Can you work these out from the drawing? Everything is in mm from the part's minimum corner. Coordinates: 2 decimals unless noted, no trailing zeros. Write each loop counter-clockwise with the first axis right and the second up, starting at its lowest first coordinate (ties: lowest second). Pieces come first, ordered by that corner, then holes. Notation, with made-up numbers: M 64,26.25 L 117,26.25 A24 cw 117,62.25 Z; hole C 89.25,9.5 d8. An arc over 180 degrees is marked long. Write item = value, one per line.
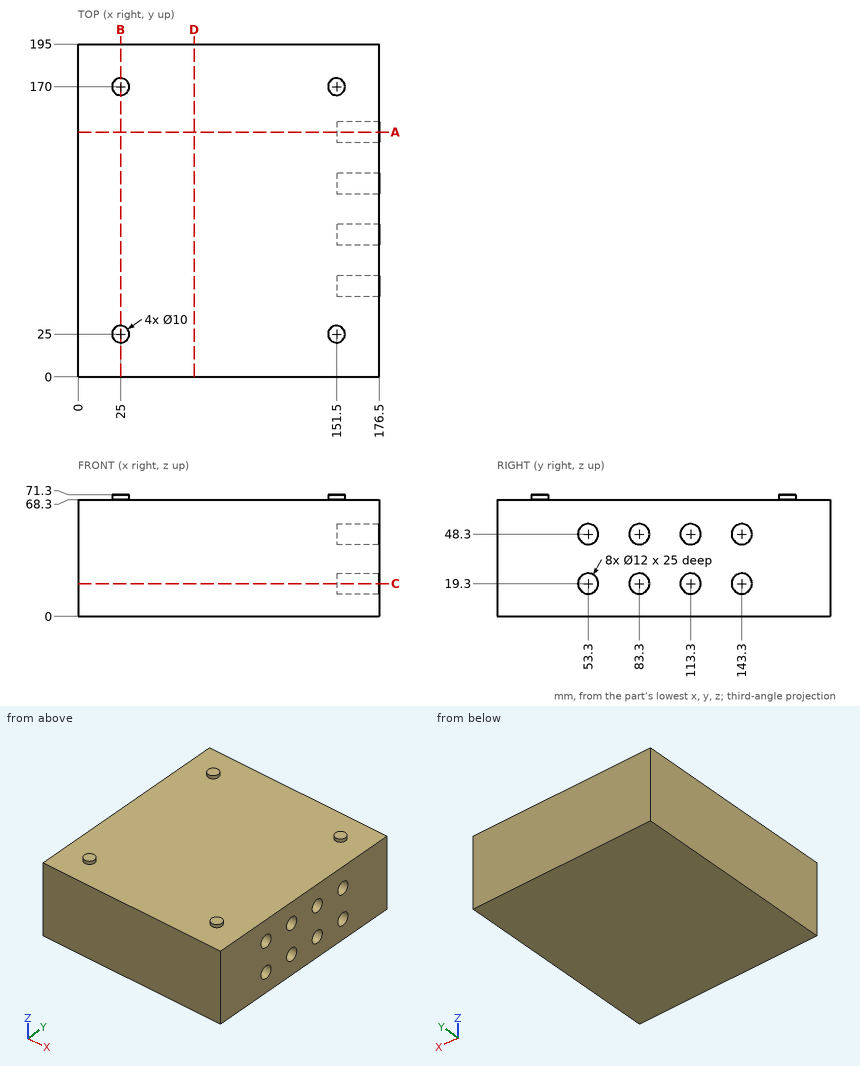
Item 1: Imagine slicing it at B-B (x = 25). Write out the boundary of the cut face in (y, z).
Numbers:
outline = M 0,0 L 195,0 L 195,68.3 L 175,68.3 L 175,71.3 L 165,71.3 L 165,68.3 L 30,68.3 L 30,71.3 L 20,71.3 L 20,68.3 L 0,68.3 Z
Item 2: Imagine slicing it at C-C (z = 19.3). Write out the boundary of the cut face in (x, y).
Numbers:
outline = M 0,0 L 176.5,0 L 176.5,47.3 L 151.5,47.3 L 151.5,59.3 L 176.5,59.3 L 176.5,77.3 L 151.5,77.3 L 151.5,89.3 L 176.5,89.3 L 176.5,107.3 L 151.5,107.3 L 151.5,119.3 L 176.5,119.3 L 176.5,137.3 L 151.5,137.3 L 151.5,149.3 L 176.5,149.3 L 176.5,195 L 0,195 Z
Item 3: Imagine slicing it at A-A (y = 143.3). Write out the boundary of the cut face in (x, z), and give its area (3 significant figures).
Numbers:
outline = M 0,0 L 176.5,0 L 176.5,13.3 L 151.5,13.3 L 151.5,25.3 L 176.5,25.3 L 176.5,42.3 L 151.5,42.3 L 151.5,54.3 L 176.5,54.3 L 176.5,68.3 L 0,68.3 Z
area = 11,500 mm²
Item 4: Imagine slicing it at D-D (x = 68). Write out the boundary of the cut face in (y, z), and give its area (3 significant figures).
Numbers:
outline = M 0,0 L 195,0 L 195,68.3 L 0,68.3 Z
area = 13,300 mm²
Item 5: I'm going to push flat-ended pins straight in: P1, Ø4, axis at y = 57, z = 31.5, coming from the -X side; P2, Ø3.5, axis at y = 143.5, z = 19.5, coming from the +X side; P3, Ø10, axis at x = 47.5, y = 82.5, coming from the +Z side. Where does each tip first touch, or does it pass through?
Numbers:
P1 = 0
P2 = 151.5
P3 = 68.3
Item 6: If I drill on line 1 along Z through (x, y) = (163.5, 143.3); line 2 along Y through (x, z) = (167, 48); line 3 along Z through (x, y) = (77, 149), over which ranges is the centre line in solid material (lowest first)?
Numbers:
line_1 = 0 to 13.3, 25.3 to 42.3, 54.3 to 68.3
line_2 = 0 to 47.31, 59.29 to 77.31, 89.29 to 107.31, 119.29 to 137.31, 149.29 to 195
line_3 = 0 to 68.3
